Autodesk Fusion 360 part; units mm, degrees
sketch "Sketch1" plane through (0, 0, 0) normal (0, 1, 0) x (1, 0, 0)
  circle A0 centre (0, 0) radius 240
  line L0 (0, 0) -> (-207.8461, -120)
  line L1 (0, 0) -> (240, 0) construction
  line L2 (0, 0) -> (207.8461, -120)
  line L3 (0, 0) -> (240, 0) construction
  line L4 (0, 0) -> (0, 240)
  line L5 (0, 240) -> (0, 180)
  line L6 (0, 180) -> (-45, 180)
  line L7 (0, 180) -> (45, 180)
  line L8 (45, 180) -> (45, 235.7435)
  line L9 (-45, 180) -> (-45, 179.9979)
  line L10 (-45, 179.9979) -> (-45, 235.7435)
  line L11 (-133.3828, -128.9701) -> (-181.6599, -156.8429)
  line L12 (-155.8846, -90) -> (-133.3846, -128.9711)
  line L13 (-155.8846, -90) -> (-178.3846, -51.0289)
  line L14 (-178.3846, -51.0289) -> (-226.6599, -78.9006)
  line L15 (178.3828, -51.0278) -> (226.6599, -78.9006)
  line L16 (155.8846, -90) -> (178.3846, -51.0289)
  line L17 (155.8846, -90) -> (133.3846, -128.9711)
  line L18 (133.3846, -128.9711) -> (181.6599, -156.8429)
  line L19 (0, 180) -> (-37.5, 180)
  line L20 (-37.5, 180) -> (-37.5, 169.5)
  circle A1 centre (-37.5, 169.5) radius 2.5
  line L21 (-37.5, 169.5) -> (-37.5, 109.5)
  line L22 (-37.5, 109.5) -> (-37.5, 49.5)
  circle A2 centre (-37.5, 109.5) radius 2.5
  circle A3 centre (-37.5, 49.5) radius 2.5
  line L23 (37.5, 109.5) -> (37.5, 49.5)
  circle A4 centre (37.5, 49.5) radius 2.5
  circle A5 centre (37.5, 109.5) radius 2.5
  line L24 (37.5, 169.5) -> (37.5, 109.5)
  circle A6 centre (37.5, 169.5) radius 2.5
  line L25 (37.5, 180) -> (37.5, 169.5)
  circle A7 centre (-165.5413, -52.274) radius 2.5
  circle A8 centre (-113.5798, -22.274) radius 2.5
  circle A9 centre (-61.6183, 7.726) radius 2.5
  circle A10 centre (-24.1183, -57.226) radius 2.5
  circle A11 centre (-76.0798, -87.226) radius 2.5
  circle A12 centre (-128.0413, -117.226) radius 2.5
  circle A13 centre (128.0413, -117.226) radius 2.5
  circle A14 centre (76.0798, -87.226) radius 2.5
  circle A15 centre (24.1183, -57.226) radius 2.5
  circle A16 centre (61.6183, 7.726) radius 2.5
  circle A17 centre (113.5798, -22.274) radius 2.5
  circle A18 centre (165.5413, -52.274) radius 2.5
  arc A19 (125.0048, -204.8751) -> (-125.0048, -204.8751) centre (0, -310.93) ccw
  line L26 (-38.4014, -152.3633) -> (-38.4014, -115.0053)
  line L27 (-38.4014, -115.0053) -> (41.5986, -115.0053)
  line L28 (41.5986, -115.0053) -> (41.5986, -152.3633)
  dimension "d90" = 480
  dimension "d91" = 150
  dimension "d92" = 30
  dimension "d100" = 60
  dimension "d101" = 45
  dimension "d102" = 45
  dimension "d104" = 360
  dimension "d105" = 37.5
  dimension "d106" = 10.5
  dimension "d107" = 5
  dimension "d108" = 60
  dimension "d109" = 60
  dimension "d110" = 5
  dimension "d111" = 5
  dimension "d113" = 360
extrude "Extrude2" add sketch "Sketch1" along normal blind 3 contours A0 L2 L4 L7 L8 L15 L16 | A0 L0 L4 L6 L10 L13 L14 L19 | A0 L0 L2 L11 L12 L17 L18 A19 L26 L27 L28
equation "d92 = 150 deg - 120 deg"
equation "d101 = ( 90 / 2 ) * 1 mm"
equation "d102 = ( 90 / 2 ) * 1 mm"
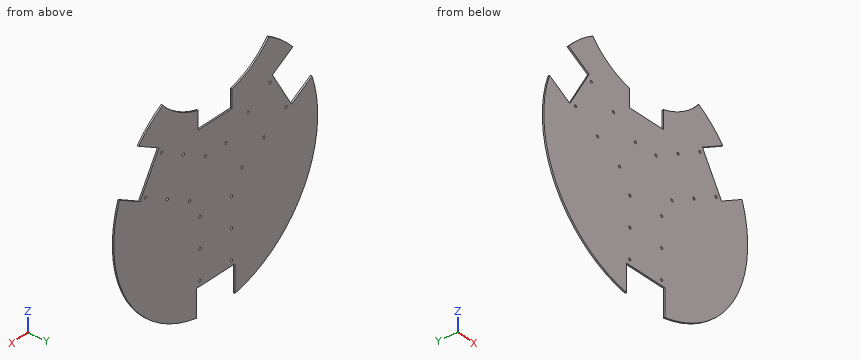
The listing builds one solid part. Answer for the finished solid, in the listing's coordinates (mm). Coordinates: 2 decimals unless noted, no trailing zeros. Write each loop counter-clockwise with the first axis right and the second up, starting at its lowest first coordinate (ties: lowest second). Pieces come first, ordered by that corner, then holes. Notation, with made-up numbers: (89, 83) - (102, 83) arc R15 cw to (102, 106) - close; hole circle Ø9 at (76, -32.5). An arc over 180 degrees is marked (long way). Answer as CSV lines item,"result".
1. Given P1, Ø1.5, axis at y = 1.5, z = 141.5, coming from the -X side; P2, Ø3, axis at x = 113.58, z = 22.27, coming from the +Y side; P3, Ø0.9, axis at x = -5.5, y = 2, coming from the -Z side; P4, Ø0.9, axis at y = 1, z = 131, coming from the +X side, each flat-ended and moving along its own axis, determine where each tip first touches the part or whether it passes through.
Computed values:
P1,"stops at x = -156.38"
P2,"passes through"
P3,"stops at z = -180"
P4,"stops at x = 137.68"
2. Find section C-C (z = -80.5). Give the vertices of the cut face in (x, y).
Computed values:
outline,"(-226.1, 0) - (226.1, 0) - (226.1, 3) - (-226.1, 3) - close"
3. Straight lines are drawn through the part: line 1 (Z direction, x = 37.5, y = 1.6); line 2 (X direction, y = 1.55, z = -169.5); line 3 (Z direction, x = -153.5, y = 1.75). For each, find the intervals that lie inside material, in ascending order. Write a range as [from, to].
Computed values:
line 1,"z = [-180, -172], [-167, -112], [-107, -52], [-47, 115.01]"
line 2,"x = [-169.91, -40], [-35, 35], [40, 169.91]"
line 3,"z = [-184.49, 94.13], [140.58, 184.49]"
4. Find section B-B (y = 0.7). Give the number of separate pieces and of enclosed holes in the cut face, plus the area to 3 significant figures.
Computed values:
separate pieces,"1"
enclosed holes,"18"
area,"146,000 mm²"
5. Find section A-A (z = -196). Give the vertices of the cut face in (x, y).
Computed values:
outline,"(-138.51, 0) - (-45, 0) - (-45, 3) - (-138.51, 3) - close; (45, 0) - (138.51, 0) - (138.51, 3) - (45, 3) - close"
